from build123d import *

# Parameters (mm, degrees)
SKETCH1_R           = 50.8
BOSS_EXTRUDE1_DEPTH = 3.175
SKETCH2_W           = 114.887790664
SKETCH2_H           = 17.737062418
CUT_EXTRUDE1_DEPTH  = 3.175
SKETCH6_R           = 1.4605
CUT_EXTRUDE2_DEPTH  = 3.175
SKETCH7_W           = 120.831003793
SKETCH7_H           = 28.526712532
CUT_EXTRUDE3_DEPTH  = 3.175
SKETCH8_W           = 6.35
SKETCH8_H           = 3.175
CUT_EXTRUDE4_DEPTH  = 3.175
SKETCH9_R           = 1.3462
CUT_EXTRUDE5_DEPTH  = 3.175


with BuildPart() as part:
    # Sketch1 → Boss-Extrude1 (new body)
    with BuildSketch(Plane(origin=(0, 0, 0), x_dir=(1, 0, 0), z_dir=(0, 1, 0))):
        Circle(SKETCH1_R)
    extrude(amount=BOSS_EXTRUDE1_DEPTH)

    # Sketch2 → Cut-Extrude1 (cut)
    with BuildSketch(Plane(origin=(0, 3.175, 0), x_dir=(1, 0, 0), z_dir=(0, 1, 0))):
        with BuildLine():
            Line((-53.141111112, 55.715142418), (61.746679552, 55.715142418))
            Line((61.746679552, 55.715142418), (61.746679552, 37.97808))
            Line((61.746679552, 37.97808), (17.466405486, 37.97808))
            add(Edge.make_bspline(
                [(17.466405486, 37.97808), (17.038082166, 26.714286782), (8.597103322, 20.19808)],
                knots=[0, 0, 0, 1, 1, 1], degree=2))
            Line((8.597103322, 20.19808), (-8.597103322, 20.19808))
            add(Edge.make_bspline(
                [(-17.466405486, 37.97808), (-17.038082166, 26.714286782), (-8.597103322, 20.19808)],
                knots=[0, 0, 0, 1, 1, 1], degree=2))
            Line((-17.466405486, 37.97808), (-53.141111112, 37.97808))
            Line((-53.141111112, 37.97808), (-53.141111112, 55.715142418))
        make_face()
        with Locations((4.30278422, -46.846611209)):
            Rectangle(SKETCH2_W, SKETCH2_H)
    extrude(amount=-CUT_EXTRUDE1_DEPTH, mode=Mode.SUBTRACT)

    # Sketch6 → Cut-Extrude2 (cut)
    with BuildSketch(Plane(origin=(0, 3.175, 0), x_dir=(1, 0, 0), z_dir=(0, 1, 0))):
        with Locations((-29.0576, 17.10182)):
            Circle(SKETCH6_R)
        with Locations((29.0576, 17.10182)):
            Circle(SKETCH6_R)
        with Locations((29.0576, -34.53638)):
            Circle(SKETCH6_R)
        with Locations((-29.0576, -34.53638)):
            Circle(SKETCH6_R)
    extrude(amount=-CUT_EXTRUDE2_DEPTH, mode=Mode.SUBTRACT)

    # Sketch7 → Cut-Extrude3 (cut)
    with BuildSketch(Plane.XZ):
        with Locations((-2.634885915, -34.53847722)):
            Rectangle(SKETCH7_W, SKETCH7_H)
    extrude(amount=-CUT_EXTRUDE3_DEPTH, mode=Mode.SUBTRACT)

    # Sketch8 → Cut-Extrude4 (cut)
    with BuildSketch(Plane.XZ):
        with Locations((-9.525, 36.39058)):
            Rectangle(SKETCH8_W, SKETCH8_H)
        with Locations((9.525, 36.39058)):
            Rectangle(SKETCH8_W, SKETCH8_H)
    extrude(amount=-CUT_EXTRUDE4_DEPTH, mode=Mode.SUBTRACT)

    # Sketch9 → Cut-Extrude5 (cut)
    with BuildSketch(Plane(origin=(0, 3.175, 0), x_dir=(1, 0, 0), z_dir=(0, 1, 0))):
        with Locations((27.725400673, 11.828091507)):
            Circle(SKETCH9_R)
        with Locations((44.133800673, 11.828091507)):
            Circle(SKETCH9_R)
        with Locations((42.533600673, -19.350408493)):
            Circle(SKETCH9_R)
        with Locations((29.325600673, -19.350408493)):
            Circle(SKETCH9_R)
    extrude(amount=-CUT_EXTRUDE5_DEPTH, mode=Mode.SUBTRACT)


solid = part.part
Verification items for the finished model (mm, model axes). A direction names the side the tool comes from. Round coordinates to 2 decimals unless told otherwise and drop trailing zeros. Order: outer loops, then holes, each group sorted by start corner. A loop starts at its lowest first (then second) coordinate and runs counter-clockwise, first axis right, second up.
1. Section check B-B on y = 1.15. State how many separate pieces and enclosed holes the cut face has, then the cut area to 3 significant figures.
Final values:
separate pieces: 1
enclosed holes: 8
area: 5,370 mm2
2. Release check for a two-part mould opening along X. For faces 4 (the cylindrical face through (-49.703, 1.565, 10.498)), 5 (the cylindrical face through (45.42, 1.61, -12.23)), 6 (the flat face through (-28, 2, -20.275)) record: +X half, -X half, draft (parallel to the pull), parting line (faces both ways), or undercut.
Final values:
face 4: -X half
face 5: undercut
face 6: draft
3. Access from +Z, -Z, +X, -X, +Y, -Y to the whole of each face (thin tool, end or side, straight path). Record for faces 1 (the flat face through (12.7, 2, 36)), 2 (the cylindrical face through (29.15, 1.61, 18.016)), 3 (the flat face through (0, 2, -20.198)).
Final values:
face 1: +Z, +Y, -Y
face 2: +Y, -Y
face 3: -Z, +Y, -Y
4. Go/stop test with flat-tipped pins: P1, Ø8, axis at x = -16, z = -9.5, coming from the -Y side; P2, Ø1, axis at x = -9, y = 1, coming from the +Z side; P3, Ø1.6, axis at y = 1, z = 36.5, coming from the +X side; P4, Ø1.5, axis at y = 0.5, z = -11, coming from the +X side. Record where each tip stops, or that it passes through.
Final values:
P1: stops at y = 0
P2: stops at z = 34.8
P3: stops at x = 36.14
P4: stops at x = 49.76
5. Thickness scan on L1, parallel to Z at x = -29.5, y = 1.65; L2, parallel to X at y = 0.2, z = -16.5; L3, parallel to X at y = 2.6, z = -17. Record the ranges inside material, lowest first.
Final values:
L1: z = -20.28 to -18.49, -15.71 to 33.14, 35.93 to 37.98
L2: x = -48.05 to -30.39, -27.73 to 27.73, 30.39 to 48.05
L3: x = -47.87 to -30.51, -27.6 to 27.6, 30.51 to 47.87
6. Section check A-A on z = 10. Record the cut outline in (x, y) (3 decimals), then the cut area to 3 significant figures.
Final values:
outline: (-49.806, 0) - (49.806, 0) - (49.806, 3.175) - (-49.806, 3.175) - close
area: 316 mm2
7. Section check C-C on x = -36. Record the cut outline in (y, z) (3 decimals).
Final values:
outline: (0, -20.275) - (3.175, -20.275) - (3.175, 35.842) - (0, 35.842) - close
